from build123d import *

# Parameters (mm, degrees)
SKETCH2_W           = 134
SKETCH2_H           = 134
SKETCH2_R           = 1.4
SKETCH2_R_2         = 1.6
BOSS_EXTRUDE2_DEPTH = 3


with BuildPart() as part:
    # Sketch2 → Boss-Extrude2 (new body)
    with BuildSketch(Plane(origin=(0, 0, 0), x_dir=(1, 0, 0), z_dir=(0, 1, 0))):
        Rectangle(SKETCH2_W, SKETCH2_H)
        with Locations((-0.080384087, -15.14345336)):
            Circle(SKETCH2_R, mode=Mode.SUBTRACT)
        with Locations((-13.830384087, -36.64345336)):
            Circle(SKETCH2_R, mode=Mode.SUBTRACT)
        with Locations((13.669615913, -36.64345336)):
            Circle(SKETCH2_R, mode=Mode.SUBTRACT)
        with Locations((-24.165395582, 44.984548377)):
            Circle(SKETCH2_R_2, mode=Mode.SUBTRACT)
        with Locations((-25.765395582, -3.315451623)):
            Circle(SKETCH2_R_2, mode=Mode.SUBTRACT)
        with Locations((26.634604418, 29.684548377)):
            Circle(SKETCH2_R_2, mode=Mode.SUBTRACT)
        with Locations((26.634604418, 1.784548377)):
            Circle(SKETCH2_R_2, mode=Mode.SUBTRACT)
        with Locations((0, 58.5)):
            Circle(SKETCH2_R_2, mode=Mode.SUBTRACT)
        with Locations((-58.5, 0)):
            Circle(SKETCH2_R_2, mode=Mode.SUBTRACT)
        with Locations((0, -58.5)):
            Circle(SKETCH2_R_2, mode=Mode.SUBTRACT)
        with Locations((58.5, 0)):
            Circle(SKETCH2_R_2, mode=Mode.SUBTRACT)
        with Locations((-37, 58.5)):
            Circle(SKETCH2_R_2, mode=Mode.SUBTRACT)
        with Locations((37, 58.5)):
            Circle(SKETCH2_R_2, mode=Mode.SUBTRACT)
        with Locations((-37, -58.5)):
            Circle(SKETCH2_R_2, mode=Mode.SUBTRACT)
        with Locations((37, -58.5)):
            Circle(SKETCH2_R_2, mode=Mode.SUBTRACT)
    extrude(amount=BOSS_EXTRUDE2_DEPTH)


solid = part.part
Can you work these out from the model? Positions are in its coordinate system, mm. Give positions to 0.01 mm unless a question says otherwise; leave off trailing zeros. Loops run counter-clockwise (first coordinate to the right, second up) from the corner with the lowest first, then second, coordinate; pieces in that order, holes last. Notation, with made-up numbers: (4.5, 26) - (29.5, 26) arc R10 ccw to (29.5, 44) - close; hole circle Ø11 at (58, -14.75). An arc over 180 degrees is marked (long way). Return JSON: item names as keys, results as strings.
1. We'd pull the mould along X, two halves only. Please class faces 1 (the face through (-23.427, 1.479, -43.565)), 2 (the face through (-1, 3, -1)), 3 (the face through (67, 1, 1)): +X half, -X half, draft (parallel to the pull), parting line (faces both ways), or undercut.
Output values:
{"face 1": "undercut", "face 2": "draft", "face 3": "+X half"}
2. I want a section at A-A on x = -58.5. Please give me the cut outline in (y, z).
Output values:
{"outline": "(0, -67) - (3, -67) - (3, -1.6) - (0, -1.6) - close; (0, 1.6) - (3, 1.6) - (3, 67) - (0, 67) - close"}
3. If I drill on line 1 (X direction, y = 1.9, z = 58.5); line 2 (X direction, y = 2.35, z = 0), over which ranges is the centre line in solid material (lowest first)?
Output values:
{"line 1": "x = -67 to -38.6, -35.4 to -1.6, 1.6 to 35.4, 38.6 to 67", "line 2": "x = -67 to -60.1, -56.9 to 56.9, 60.1 to 67"}
4. I want a section at C-C on x = -37. Please give me the cut outline in (y, z), and give its area (3 significant figures).
Output values:
{"outline": "(0, -67) - (3, -67) - (3, -60.1) - (0, -60.1) - close; (0, -56.9) - (3, -56.9) - (3, 56.9) - (0, 56.9) - close; (0, 60.1) - (3, 60.1) - (3, 67) - (0, 67) - close", "area": "383 mm²"}
5. I want a section at B-B on z = 58.5. Please give me the cut outline in (x, y).
Output values:
{"outline": "(-67, 0) - (-38.6, 0) - (-38.6, 3) - (-67, 3) - close; (-35.4, 0) - (-1.6, 0) - (-1.6, 3) - (-35.4, 3) - close; (1.6, 0) - (35.4, 0) - (35.4, 3) - (1.6, 3) - close; (38.6, 0) - (67, 0) - (67, 3) - (38.6, 3) - close"}
6. I'm going to push a flat-ended pin straight in: pin 1 Ø1.9 at (x, z) = (-37, 58.5) entering from -Y. Where does the tip first touch, or does it pass through?
Output values:
{"pin 1": "passes through"}
